The listing builds one solid part. Answer for the finished solid, in the listing's coordinates (mm). Face numbers are marked on the shaded views. A direction names the side the tool comes from. Round coordinates to 2 decimals unless told otherwise and drop trailing zeros. Loops run counter-clockwise (first coordinate to the right, second up) from the corner with the lowest first, then second, coordinate; pieces in that order, holes last. Notation, with made-up numbers: M -4.75,21 L 37.25,21 A38 cw 37.25,60 Z; hole C -33,15 d9. An arc over 180 degrees is marked long. Answer as a JSON object with one key per item and string values.
```python
from build123d import *

# Parameters (mm, degrees)
F1_DEPTH  = 33
F3_W      = 1.8808413297
F3_H      = 18.471846357
F4_DEPTH  = 33
F5_R      = 2
F6_DEPTH  = 3
F7_W      = 18.471846357
F7_H      = 5
F8_DEPTH  = 5
F9_DEPTH  = 5
F2_R      = 2.125
F10_DEPTH = 25


# Not quite as in the source:
# - a feature names something its author has since deleted; it is built from what else it names


with BuildPart() as f1:
    # F0 (on Top) → F1 (new body)
    with BuildSketch(Plane.XY):
        with BuildLine():
            ThreePointArc((-23.401635828, 2.1478921234), (-23.2315061267, 3.5421918479), (-22.9783775489, 4.9238364331))
            Line((-22.9783775489, 4.9238364331), (-32.5732277849, 4.9238364331))
            Line((-32.5732277849, 4.9238364331), (-32.5732277849, 2.1478921234))
            Line((-32.5732277849, 2.1478921234), (-23.401635828, 2.1478921234))
        make_face()
        with BuildLine():
            Line((-32.5732277849, -5.0761635669), (-22.9452078535, -5.0761635669))
            ThreePointArc((-22.9452078535, -5.0761635669), (-23.2124017724, -3.6652972535), (-23.3929275249, -2.2407458164))
            Line((-23.3929275249, -2.2407458164), (-32.5732277849, -2.2407458164))
            Line((-32.5732277849, -2.2407458164), (-32.5732277849, -5.0761635669))
        make_face()
        with BuildLine():
            ThreePointArc((-22.9452078535, -5.0761635669), (2.55319559, -23.3608902287), (23.5, 0))
            ThreePointArc((23.5, 0), (2.4756946097, 23.3692305436), (-22.9783775489, 4.9238364331))
            Line((-22.9783775489, 4.9238364331), (-17.5732277849, 4.9238364331))
            ThreePointArc((-17.5732277849, 4.9238364331), (2.4850646798, 18.080015308), (18.25, 0))
            ThreePointArc((18.25, 0), (2.4850646798, -18.080015308), (-17.5732277849, -4.9238364331))
            Line((-17.5732277849, -4.9238364331), (-17.5732277849, -5.0761635669))
            Line((-17.5732277849, -5.0761635669), (-22.9452078535, -5.0761635669))
        make_face()
        with BuildLine():
            Line((-17.5732277849, 4.9238364331), (-22.9783775489, 4.9238364331))
            ThreePointArc((-22.9783775489, 4.9238364331), (-23.2315061267, 3.5421918479), (-23.401635828, 2.1478921234))
            Line((-23.401635828, 2.1478921234), (-18.1231636153, 2.1478921234))
            ThreePointArc((-18.1231636153, 2.1478921234), (-17.9020824613, 3.5465396584), (-17.5732277849, 4.9238364331))
        make_face()
        with BuildLine():
            ThreePointArc((-23.3929275249, -2.2407458164), (-23.2124017724, -3.6652972535), (-22.9452078535, -5.0761635669))
            Line((-22.9452078535, -5.0761635669), (-17.5732277849, -5.0761635669))
            Line((-17.5732277849, -5.0761635669), (-17.5732277849, -4.9238364331))
            ThreePointArc((-17.5732277849, -4.9238364331), (-17.9020824613, -3.5465396584), (-18.1231636153, -2.1478921234))
            Line((-18.1231636153, -2.1478921234), (-18.1231636153, -2.2407458164))
            Line((-18.1231636153, -2.2407458164), (-23.3929275249, -2.2407458164))
        make_face()
    extrude(amount=F1_DEPTH)

    # F3 (on Top) → F4 (join)
    with BuildSketch(Plane.XY):
        with Locations((22.5681019947, 0.0180900097)):
            Rectangle(F3_W, F3_H)
    extrude(amount=F4_DEPTH)

    # F5 (on face) → F6 (cut)
    with BuildSketch(Plane.XY.offset(33)):
        with Locations((0, 20.875)):
            Circle(F5_R)
        with Locations((0, -20.875)):
            Circle(F5_R)
    extrude(amount=-F6_DEPTH, mode=Mode.SUBTRACT)

    # F7 (on face) → F8 (cut)
    with BuildSketch(Plane.YZ.offset(23.5085226595)):
        with Locations((0.0180900097, 30.5)):
            Rectangle(F7_W, F7_H)
    extrude(amount=-F8_DEPTH, mode=Mode.SUBTRACT)

    # F7 (on face) → F9 (join)
    with BuildSketch(Plane.YZ.offset(23.5085226595)):
        with Locations((0.0180900097, 2.5)):
            Rectangle(F7_W, F7_H)
    extrude(amount=F9_DEPTH)

    # F2 (on face) → F10 (cut)
    with BuildSketch(Plane.XZ.offset(5.0761635669)):
        with Locations((-27.5732277849, 16.5)):
            Circle(F2_R)
    extrude(amount=-F10_DEPTH, mode=Mode.SUBTRACT)


solid = f1.part
```
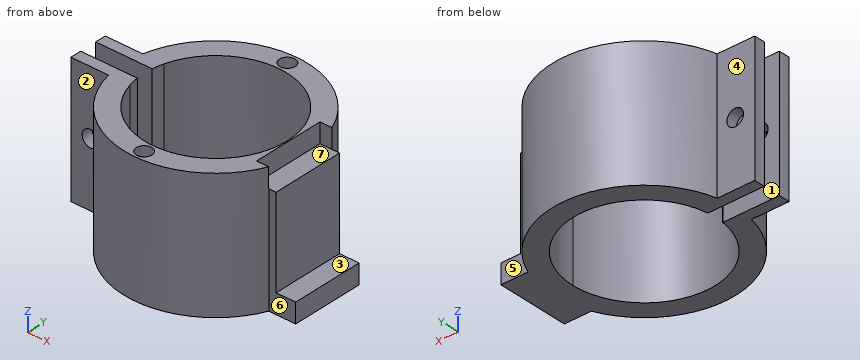
Item 1: The part is cut by section D-D (x = -27). Give the vertices of the cut face in (y, z), then the cut area to 3 significant figures.
Values follow:
{"outline": "M -5.08,0 L -2.24,0 L -2.24,14.45 L -5.08,14.45 Z; M -5.08,18.55 L -2.24,18.55 L -2.24,33 L -5.08,33 Z; M 2.15,0 L 4.92,0 L 4.92,14.45 L 2.15,14.45 Z; M 2.15,18.55 L 4.92,18.55 L 4.92,33 L 2.15,33 Z", "area": "162 mm^2"}
Item 2: Straight lines are drawn through the part: line 1 (Y direction, x = 0, z = 32) (3 decimals); line 2 (Y direction, x = -30, z = 20); line 3 (Y direction, x = 0, z = 20). For each, find the intervals that lie inside material, in ascending order.
Values follow:
{"line 1": "-23.5 to -22.875, -18.875 to -18.25, 18.25 to 18.875, 22.875 to 23.5", "line 2": "-5.08 to -2.24, 2.15 to 4.92", "line 3": "-23.5 to -18.25, 18.25 to 23.5"}
Item 3: The part is cut by section B-B (z = 16.5). Give the number of separate pieces and of enclosed holes in the cut face, then the cut area to 3 significant figures.
Values follow:
{"separate pieces": "3", "enclosed holes": "0", "area": "706 mm^2"}
Item 4: The part is cut by section A-A (x = 0). Give the vertices of the cut face in (y, z) (3 decimals).
Values follow:
{"outline": "M -23.5,0 L -18.25,0 L -18.25,33 L -18.875,33 L -18.875,30 L -22.875,30 L -22.875,33 L -23.5,33 Z; M 18.25,0 L 23.5,0 L 23.5,33 L 22.875,33 L 22.875,30 L 18.875,30 L 18.875,33 L 18.25,33 Z"}
Item 5: The part is cut by section C-C (y = 10). Give the vertices of the cut face in (x, z).
Values follow:
{"outline": "M -21.27,0 L -15.27,0 L -15.27,33 L -21.27,33 Z; M 15.27,0 L 21.27,0 L 21.27,33 L 15.27,33 Z"}
Item 6: Flat-ended cylindrical pins translate along their axes: P1, Ø3, axis at y = 14, z = 8, coming from the -X side; P2, Ø12, axis at y = -16.5, z = 7, coming from the +X side; P3, Ø2.5, axis at x = -27.57, z = 16.5, coming from the -Y side; P4, Ø3, axis at x = -16, z = 28.5, coming from the +Y side. Find the tip coordinate at first contact, or state that the pin passes through.
Values follow:
{"P1": "x = -19.9", "P2": "x = 21.02", "P3": "through", "P4": "y = 18.49"}
Item 7: Determine the mould class of the marked faces 5, 6 and 7 for opening direction Y: released by +Y, released by -Y, zero draft, split by the parting line, or undercut.
Values follow:
{"face 5": "released by +Y", "face 6": "released by -Y", "face 7": "undercut"}
Item 8: Which of the six approach directions +Z, -Z, +X, -X, +Y, -Y give full straight-line access (tool end or side, diameter ignored) to the marked faces 1, 2, 3 and 4?
Values follow:
{"face 1": "+Z, -Z, -X", "face 2": "+Z, -Z, -X, -Y", "face 3": "+Z, +X, +Y, -Y", "face 4": "+Z, -Z, -X, +Y"}
